Can you work these out from the model? Positions are in its coordinate system, mm. Coordinates: 2 decimals unless noted, no trailing zeros. Loops run counter-clockwise (first coordinate to the right, second up) from the corner with the lowest first, then second, coordinate; pieces in that order, holes last.
```python
from build123d import *

# Parameters (mm, degrees)
SKETCH1_W                    = 7.112
SKETCH1_H                    = 1.5875
F_36_0_1065_DIAMETER_HOLE1_D = 2.7051
SCREW_PASSTHROUGHS_COUNT     = 12


with BuildPart() as part:
    # Sketch1 → Main (revolve)
    with BuildSketch(Plane.XY):
        with Locations((-41.656, 0.79375)):
            Rectangle(SKETCH1_W, SKETCH1_H)
    revolve(axis=Axis((0, 55, 0), (0, -1, 0)))

    # #36 (0.1065) Diameter Hole1 (through all)
    with Locations(Plane(origin=(0, 0, 0), x_dir=(-1, 0, 0), z_dir=(0, -1, 0))):
        with Locations((41.656, 0)):
            f_36_0_1065_diameter_hole1 = Hole(F_36_0_1065_DIAMETER_HOLE1_D / 2)

    # Screw Passthroughs: #36 (0.1065) Diameter Hole1 ×12 about axis
    screw_passthroughs_axis = Axis((0, 0, 0), (0, 1, 0))
    for i in range(1, SCREW_PASSTHROUGHS_COUNT):
        add(f_36_0_1065_diameter_hole1.rotate(screw_passthroughs_axis, i * 360 / SCREW_PASSTHROUGHS_COUNT), mode=Mode.SUBTRACT)


solid = part.part
```
Item 1: Suppose I cut it at A-A, the plane x = 0. Please give me the cut outline in (y, z), plus the area to 3 significant figures.
Results are:
outline: (0, -45.21) - (1.59, -45.21) - (1.59, -43.01) - (0, -43.01) - close; (0, -40.3) - (1.59, -40.3) - (1.59, -38.1) - (0, -38.1) - close; (0, 38.1) - (1.59, 38.1) - (1.59, 40.3) - (0, 40.3) - close; (0, 43.01) - (1.59, 43.01) - (1.59, 45.21) - (0, 45.21) - close
area: 14.0 mm2
Item 2: Suppose I cut it at B-B, the plane z = 0. Please give me the cut outline in (x, y), plus the area to 3 significant figures.
Results are:
outline: (-45.21, 0) - (-43.01, 0) - (-43.01, 1.59) - (-45.21, 1.59) - close; (-40.3, 0) - (-38.1, 0) - (-38.1, 1.59) - (-40.3, 1.59) - close; (38.1, 0) - (40.3, 0) - (40.3, 1.59) - (38.1, 1.59) - close; (43.01, 0) - (45.21, 0) - (45.21, 1.59) - (43.01, 1.59) - close
area: 14.0 mm2
Item 3: Suppose I cut it at D-D, the plane z = 29. Please give me the cut outline in (x, y).
Results are:
outline: (-34.69, 0) - (-24.71, 0) - (-24.71, 1.59) - (-34.69, 1.59) - close; (24.71, 0) - (34.69, 0) - (34.69, 1.59) - (24.71, 1.59) - close
Item 4: I need wall thicknesses on line 1 along X through (y, z) = (1.4, -20.5); line 2 along Z through (x, y) = (20, 1.55); line 3 along X through (y, z) = (0.5, -26.5). Which ranges of each line are inside material? Lowest first, please.
Results are:
line 1: x = -40.3 to -37.39, -34.76 to -32.11, 32.11 to 34.76, 37.39 to 40.3
line 2: z = -40.55 to -37.14, -35.01 to -32.43, 32.43 to 35.01, 37.14 to 40.55
line 3: x = -36.63 to -27.37, 27.37 to 36.63
Item 5: Suppose I cut it at C-C, the plane y = 1.15. Count the separate pieces of the cut face and the enclosed holes in it, plus the area to 3 significant figures.
Results are:
separate pieces: 1
enclosed holes: 13
area: 1,790 mm2
Item 6: We'd pull the mould along Z, two halves only. Please class faces 1 (the face through (-36.48, 0.8, -22.12)), 2 (the face through (37, 1.587, 10)), 3 (the face through (9.801, 0.805, 44.137)): +Z half, -Z half, draft (parallel to the pull), parting line (faces both ways), or undercut.
Results are:
face 1: undercut
face 2: draft
face 3: parting line
